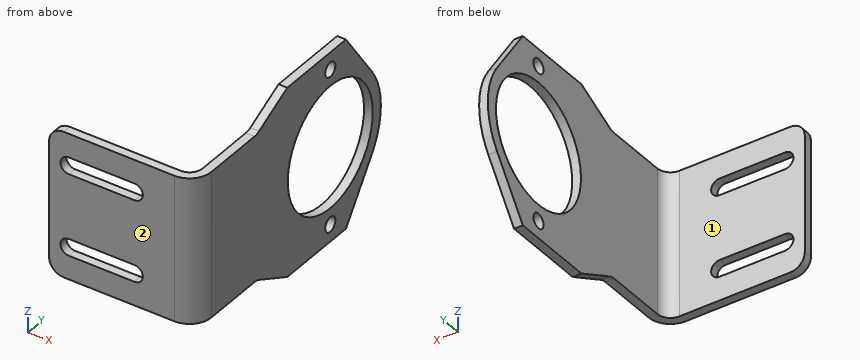
```python
from build123d import *

# Parameters (mm, degrees)
BASE_FLANGE1_DEPTH      = 65
SKETCH6_R               = 42
SKETCH6_R_2             = 5
CUT_EXTRUDE1_DEPTH      = 10
CUT_EXTRUDE2_DEPTH      = 219.477115506
CUT_EXTRUDE2_DEPTH_BACK = 219.477115506
SKETCH8_OUTSIDE_W       = 181.156
SKETCH8_OUTSIDE_H       = 233.656
CUT_EXTRUDE3_DEPTH      = 10
BREAK_CORNER1_START     = -6
BREAK_CORNER1_DEPTH     = 6
BREAK_CORNER1_2_DEPTH   = 6


# Read off the part's stored shape, not the designer's step: Break-Corner1
# Sheet-metal steps are written as plain solids
with BuildPart() as part:
    # Sketch1 → Base-Flange1 (new, symmetric)
    with BuildSketch(Plane.XY):
        with BuildLine():
            Line((-101, 0), (-15, 0))
            ThreePointArc((-15, 0), (-4.393398282, 4.393398282), (0, 15))
            Line((0, 15), (0, 182.5))
            Line((0, 182.5), (-6, 182.5))
            Line((-6, 182.5), (-6, 15))
            ThreePointArc((-6, 15), (-8.636038969, 8.636038969), (-15, 6))
            Line((-15, 6), (-101, 6))
            Line((-101, 6), (-101, 0))
        make_face()
    extrude(amount=BASE_FLANGE1_DEPTH, both=True)

    # Sketch6 → Cut-Extrude1 (cut)
    with BuildSketch(Plane.ZY.offset(6)):
        with Locations((0, 132.5)):
            Circle(SKETCH6_R)
        with Locations((-53.2, 132.5)):
            Circle(SKETCH6_R_2)
        with Locations((53.2, 132.5)):
            Circle(SKETCH6_R_2)
    extrude(amount=-CUT_EXTRUDE1_DEPTH, mode=Mode.SUBTRACT)

    # Sketch8 outside → Cut-Extrude2 (cut, two sides: drawn at the far end of the back side and taken through both)
    with BuildSketch(Plane(origin=(0, 0, 0), x_dir=(0, 0, -1), z_dir=(1, 0, 0)).offset(-CUT_EXTRUDE2_DEPTH_BACK)):
        with Locations((0, 91.25)):
            Rectangle(SKETCH8_OUTSIDE_W, SKETCH8_OUTSIDE_H)
        with BuildLine():
            Line((50, 0), (50, 60))
            Line((50, 60), (65, 90))
            Line((65, 90), (65, 148))
            Line((65, 148), (28.697915295, 173.444226183))
            ThreePointArc((28.697915295, 173.444226183), (0, 182.5), (-28.697915295, 173.444226183))
            Line((-28.697915295, 173.444226183), (-65, 148))
            Line((-65, 148), (-65, 90))
            Line((-65, 90), (-50, 60))
            Line((-50, 60), (-50, 0))
            Line((-50, 0), (50, 0))
        make_face(mode=Mode.SUBTRACT)
    extrude(amount=CUT_EXTRUDE2_DEPTH + CUT_EXTRUDE2_DEPTH_BACK, mode=Mode.SUBTRACT)

    # Sketch7 → Cut-Extrude3 (cut)
    with BuildSketch(Plane(origin=(0, 6, 0), x_dir=(1, 0, 0), z_dir=(0, 1, 0))):
        with BuildLine():
            Line((-42.45, 22.2), (-87.45, 22.2))
            ThreePointArc((-87.45, 22.2), (-93.2, 27.95), (-87.45, 33.7))
            Line((-87.45, 33.7), (-42.45, 33.7))
            ThreePointArc((-42.45, 33.7), (-36.7, 27.95), (-42.45, 22.2))
        make_face()
        with BuildLine():
            Line((-42.45, -33.8), (-87.45, -33.8))
            ThreePointArc((-87.45, -33.8), (-93.2, -28.05), (-87.45, -22.3))
            Line((-87.45, -22.3), (-42.45, -22.3))
            ThreePointArc((-42.45, -22.3), (-36.7, -28.05), (-42.45, -33.8))
        make_face()
    extrude(amount=-CUT_EXTRUDE3_DEPTH, mode=Mode.SUBTRACT)

    # Break-Corner1 outline → Break-Corner1 (add)
    with BuildSketch(Plane.YZ.offset(BREAK_CORNER1_START)):
        with BuildLine():
            Line((60, 50), (62.11145618, 51.05572809))
            ThreePointArc((62.11145618, 51.05572809), (59.936849431, 50.267510105), (57.639320225, 50))
            Line((57.639320225, 50), (60, 50))
        make_face()
        with BuildLine():
            Line((60, -50), (57.639320225, -50))
            ThreePointArc((57.639320225, -50), (59.936849431, -50.267510105), (62.11145618, -51.05572809))
            Line((62.11145618, -51.05572809), (60, -50))
        make_face()
    extrude(amount=BREAK_CORNER1_DEPTH)

    # Break-Corner1 2 outline → Break-Corner1 2 (cut)
    with BuildSketch(Plane(origin=(0, 0, 0), x_dir=(1, 0, 0), z_dir=(0, 1, 0))):
        with BuildLine():
            Line((-101, -50), (-91, -50))
            ThreePointArc((-91, -50), (-98.071067812, -47.071067812), (-101, -40))
            Line((-101, -40), (-101, -50))
        make_face()
        with BuildLine():
            Line((-101, 50), (-101, 40))
            ThreePointArc((-101, 40), (-98.071067812, 47.071067812), (-91, 50))
            Line((-91, 50), (-101, 50))
        make_face()
    extrude(amount=BREAK_CORNER1_2_DEPTH, mode=Mode.SUBTRACT)


solid = part.part
```
CAD build for the part. Positions are in the model's coordinates, mm. Face numbers are marked on the shaded views. A direction names the side the tool comes from. Round coordinates to 2 decimals unless told otherwise and drop trailing zeros. Order: outer loops, then holes, each group sorted by start corner. A loop starts at its lowest first (then second) coordinate and runs counter-clockwise, first axis right, second up.
Item 1: Tool access for the marked faces 1 and 2: list every direction of +Z, -Z, +X, -X, +Y, -Y with a clear straight run to the whole face (end or side of a thin tool).
Item 2: Saw through at D-D on y = 108. Write the cut outline in (x, z).
Item 3: Saw through at C-C on z = 0. Write the cut outline in (x, y), then the cut area to 3 significant figures.
Item 4: Pin check, flat tips, straight feed: pin 1 (6.5 mm diameter, centred on x = -59.5, y = 3, fed in from -Z); pin 2 (5 mm diameter, centred on x = -75, y = 4.5, fed in from +Z); pin 3 (12 mm diameter, centred on x = -75, z = 50.5, fed in from +Y); pin 4 (13 mm diameter, centred on y = 132.5, z = -53.2, fed in from +X). Stop position of each tip, or through.
Item 5: Probe line 1 along Z through (x, y) = (-1, 132); line 2 along Y through (x, z) = (-89, 1); line 3 along X through (y, z) = (163, -36.5). List the from-to ranges inside material, lowest first.
Item 6: Saw through at A-A on x = -79. Write the cut outline in (y, z), then the cut area to 3 significant figures.
Item 7: Saw through at B-B on y = 132.5. Write the cut outline in (x, z), then the cut area to 3 significant figures.
Reported:
1. face 1: +Z, -Z, -X, +Y
1. face 2: +Z, -Z, +X, -X, -Y
2. outline: (-6, -65) - (0, -65) - (0, -34.11) - (-6, -34.11) - close; (-6, 34.11) - (0, 34.11) - (0, 65) - (-6, 65) - close
3. outline: (-101, 0) - (-15, 0) arc R15 ccw to (0, 15) - (0, 90.5) - (-6, 90.5) - (-6, 15) arc R9 cw to (-15, 6) - (-101, 6) - close; (-6, 174.5) - (0, 174.5) - (0, 182.5) - (-6, 182.5) - close
3. area: 1,130 mm2
4. pin 1: stops at z = -50
4. pin 2: stops at z = 50
4. pin 3: stops at y = 6
4. pin 4: stops at x = 0
5. line 1: z = -65 to -58.17, -48.23 to -42, 42 to 48.23, 58.17 to 65
5. line 2: y = 0 to 6
5. line 3: x = -6 to 0
6. outline: (0, -50) - (6, -50) - (6, -33.7) - (0, -33.7) - close; (0, -22.2) - (6, -22.2) - (6, 22.3) - (0, 22.3) - close; (0, 33.8) - (6, 33.8) - (6, 50) - (0, 50) - close
6. area: 462 mm2
7. outline: (-6, -65) - (0, -65) - (0, -58.2) - (-6, -58.2) - close; (-6, -48.2) - (0, -48.2) - (0, -42) - (-6, -42) - close; (-6, 42) - (0, 42) - (0, 48.2) - (-6, 48.2) - close; (-6, 58.2) - (0, 58.2) - (0, 65) - (-6, 65) - close
7. area: 156 mm2
